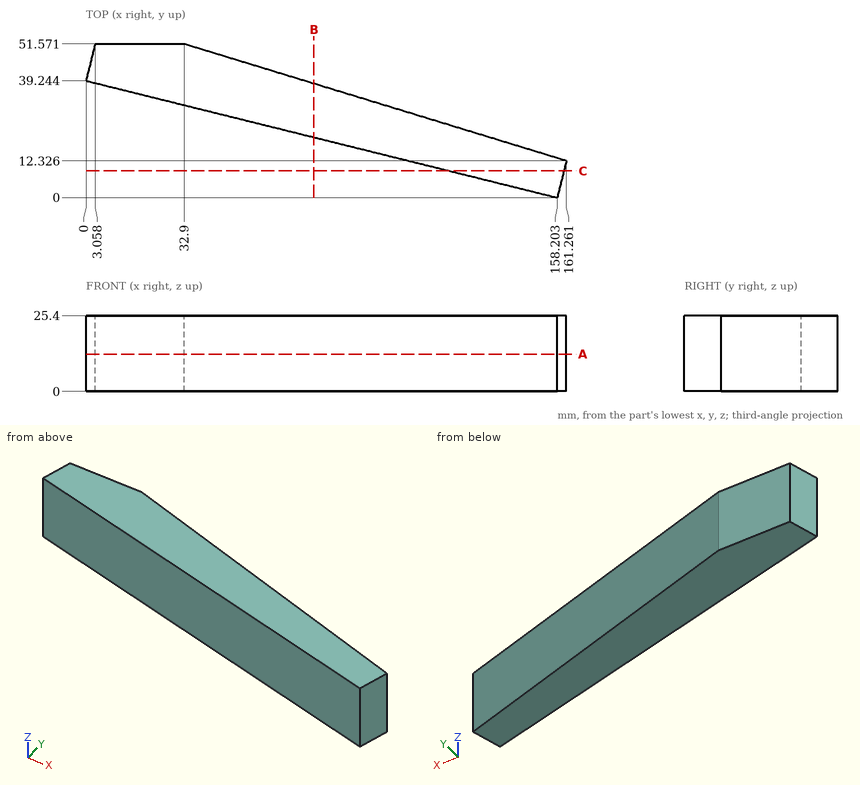
Here's the drawing with two shaded views (mm, measured from the low corner). I have some questions. Give positions to 0.01 mm unless a question says otherwise; leave off trailing zeros. Loops run counter-clockwise (first coordinate to the right, second up) from the corner with the lowest first, then second, coordinate; pieces in that order, holes last. Notation, with made-up numbers: (-37, 71) -> (10, 71) arc R18 cw to (10, 101) -> close; hole circle Ø8 at (-26.5, 67.25). An arc over 180 degrees is marked (long way). Answer as a JSON object with one key per item and string values. Group by question number.
Item 1: Imagine slicing it at B-B on x = 76.5. Write out the boundary of the cut face in (y, z).
Item 2: Imagine slicing it at C-C on y = 9. Write out the boundary of the cut face in (x, z), then the cut area to 3 significant figures.
Item 3: I need wall thicknesses on L1, parallel to Y at x = 79, z = 1 (1 decimal); L2, parallel to Y at x = 119.5, z = 11.75 (1 decimal). Which ranges of each line are inside material? Lowest first, please.
Item 4: Will these pins go through, and if not, where does the flat tip stop? pin 1 (10 mm diameter, centred on x = 51.5, z = 9.5, fed in from +Y); pin 2 (1 mm diameter, centred on x = 76, z = 19, fed in from +Y); pin 3 (1.5 mm diameter, centred on x = 40.5, z = 21, fed in from -Y).
Item 5: Imagine slicing it at A-A on z = 12.5. Write out the boundary of the cut face in (x, y) (1 decimal).
Answer list:
{
 "1": {"outline": "(20.27, 0) -> (38.24, 0) -> (38.24, 25.4) -> (20.27, 25.4) -> close"},
 "2": {"outline": "(121.92, 0) -> (160.44, 0) -> (160.44, 25.4) -> (121.92, 25.4) -> close", "area": "978 mm2"},
 "3": {"L1": "y = 19.6 to 37.5", "L2": "y = 9.6 to 25.1"},
 "4": {"pin 1": "stops at y = 47.41", "pin 2": "stops at y = 38.55", "pin 3": "stops at y = 29.01"},
 "5": {"outline": "(0, 39.2) -> (158.2, 0) -> (161.3, 12.3) -> (32.9, 51.6) -> (3.1, 51.6) -> close"}
}
